Work out the finished part from the listing and answer in its coordinate system (mm). A direction names the side the tool comes from. Give positions to 0.01 mm unless a question says otherwise; leave off trailing zeros. Loops run counter-clockwise (first coordinate to the right, second up) from the corner with the lowest first, then second, coordinate; pieces in that order, holes last. Notation, with made-up numbers: (6, -39.5) - (31, -39.5) arc R22 cw to (31, -14.5) - close; hole circle Ø5 at (-35, 73.25). An arc over 180 degrees is marked (long way). One line per question, with ' | ' between items.
from build123d import *

# Parameters (mm, degrees)
CROQUIS1_R                 = 30.5
SALIENTE_EXTRUIR1_DEPTH    = 2.4
CROQUIS2_R                 = 2
CORTAR_EXTRUIR1_DEPTH      = 4
CORTAR_EXTRUIR3_START      = -4
CORTAR_EXTRUIR3_DEPTH      = 4
CORTAR_EXTRUIR5_START      = -4
CORTAR_EXTRUIR5_DEPTH      = 4
CORTAR_EXTRUIR6_DEPTH      = 10
CROQUIS10_R                = 2.5
CORTAR_EXTRUIR7_DEPTH      = 3
CORTAR_EXTRUIR8_DEPTH      = 44.200231628
CORTAR_EXTRUIR8_DEPTH_BACK = 44.200231628
CORTAR_EXTRUIR9_START      = -10
CORTAR_EXTRUIR9_DEPTH      = 10
REDONDEO1_R                = 1
CORTAR_EXTRUIR10_DEPTH     = 3


with BuildPart() as part:
    # Croquis1 → Saliente-Extruir1 (new body)
    with BuildSketch(Plane(origin=(0, 0, 0), x_dir=(1, 0, 0), z_dir=(0, 1, 0))):
        with Locations(Location((0, 0, 0), (0, 0, 270))):
            Circle(CROQUIS1_R)
    extrude(amount=SALIENTE_EXTRUIR1_DEPTH)

    # Croquis2 → Cortar-Extruir1 (cut)
    with BuildSketch(Plane(origin=(0, 2.4, 0), x_dir=(1, 0, 0), z_dir=(0, 1, 0))):
        with Locations(Location((0, 0, 0), (0, 0, 270))):
            Circle(CROQUIS2_R)
    extrude(amount=-CORTAR_EXTRUIR1_DEPTH, mode=Mode.SUBTRACT)

    # Croquis5 → Cortar-Extruir3 (cut)
    with BuildSketch(Plane(origin=(0, 2.4, 0), x_dir=(1, 0, 0), z_dir=(0, 1, 0)).offset(CORTAR_EXTRUIR3_START)):
        with BuildLine():
            Line((28.814059068, 5), (30.087372767, 5))
            ThreePointArc((30.087372767, 5), (29.556634924, 7.526973624), (28.814059068, 10))
            Line((28.814059068, 10), (24.814059068, 10))
            Line((24.814059068, 10), (24.814059068, 5))
            Line((24.814059068, 5), (28.814059068, 5))
        make_face()
        with BuildLine():
            Line((30.087372767, -5), (28.814059068, -5))
            Line((28.814059068, -5), (24.814059068, -5))
            Line((24.814059068, -5), (24.814059068, -10))
            Line((24.814059068, -10), (28.814059068, -10))
            ThreePointArc((28.814059068, -10), (29.556634924, -7.526973624), (30.087372767, -5))
        make_face()
        with BuildLine():
            Line((-24.814059068, 5), (-24.814059068, 10))
            Line((-24.814059068, 10), (-28.814059068, 10))
            ThreePointArc((-28.814059068, 10), (-29.556634924, 7.526973624), (-30.087372767, 5))
            Line((-30.087372767, 5), (-28.814059068, 5))
            Line((-28.814059068, 5), (-24.814059068, 5))
        make_face()
        with BuildLine():
            Line((-28.814059068, -10), (-24.814059068, -10))
            Line((-24.814059068, -10), (-24.814059068, -5))
            Line((-24.814059068, -5), (-28.814059068, -5))
            Line((-28.814059068, -5), (-30.087372767, -5))
            ThreePointArc((-30.087372767, -5), (-29.556634924, -7.526973624), (-28.814059068, -10))
        make_face()
    extrude(amount=CORTAR_EXTRUIR3_DEPTH, mode=Mode.SUBTRACT)

    # Croquis7 → Cortar-Extruir5 (cut)
    with BuildSketch(Plane(origin=(0, 2.4, 0), x_dir=(1, 0, 0), z_dir=(0, 1, 0)).offset(CORTAR_EXTRUIR5_START)):
        Polygon((1.428390211, 22.411430151), (-0.869743118, 20.483067322), (2.34419493, 16.652845106), (4.642328259, 18.581207935), align=None)
        with BuildLine():
            Line((-24.814059068, -10), (-28.814059068, -10))
            ThreePointArc((-28.814059068, -10), (0, -30.5), (28.814059068, -10))
            Line((28.814059068, -10), (24.814059068, -10))
            add(Edge.make_bspline(
                [(24.814059068, -10), (22.863263717, -9.657344338), (20.984021298, -8.980450277), (19.168992989, -8.065339906)],
                knots=[0, 0, 0, 0, 0.087850084, 0.087850084, 0.087850084, 0.087850084], degree=3))
            Line((19.168992989, -8.065339906), (11.455541673, 1.127193412))
            Line((11.455541673, 1.127193412), (9.248678515, -0.72458465))
            add(Edge.make_bspline(
                [(9.248678515, -0.72458465), (4.033234859, 4.116641048), (-0.646914404, 9.508508747), (-5.04935939, 12.080675515)],
                knots=[0.258799312, 0.258799312, 0.258799312, 0.258799312, 0.546435258, 0.546435258, 0.546435258, 0.546435258], degree=3))
            Line((-5.04935939, 12.080675515), (-0.757422911, 15.682037831))
            Line((-0.757422911, 15.682037831), (-7.828086618, 24.108526705))
            Line((-7.828086618, 24.108526705), (-17.020619935, 16.395075389))
            Line((-17.020619935, 16.395075389), (-13.66601447, 12.397212273))
            add(Edge.make_bspline(
                [(-13.66601447, 12.397212273), (-17.403465693, 9.897923685), (-21.056529869, 3.255841362), (-24.814059068, -10)],
                knots=[0.740637404, 0.740637404, 0.740637404, 0.740637404, 1, 1, 1, 1], degree=3))
        make_face()
        Polygon((14.685884661, 6.611763511), (12.387751331, 4.683400682), (15.60168938, 0.853178467), (17.899822709, 2.781541296), align=None)
    extrude(amount=CORTAR_EXTRUIR5_DEPTH, mode=Mode.SUBTRACT)

    # Croquis9 → Cortar-Extruir6 (cut)
    with BuildSketch(Plane(origin=(0, 2.4, 0), x_dir=(1, 0, 0), z_dir=(0, 1, 0))):
        Polygon((7.971418181, 14.613753061), (5.673284852, 12.685390231), (8.887222901, 8.855168016), (11.18535623, 10.783530845), align=None)
    extrude(amount=-CORTAR_EXTRUIR6_DEPTH, mode=Mode.SUBTRACT)

    # Croquis10 → Cortar-Extruir7 (cut)
    with BuildSketch(Plane(origin=(0, 2.4, 0), x_dir=(1, 0, 0), z_dir=(0, 1, 0))):
        with Locations(Location((12, 16, 0), (0, 0, 270))):
            Circle(CROQUIS10_R)
    extrude(amount=-CORTAR_EXTRUIR7_DEPTH, mode=Mode.SUBTRACT)

    # Croquis11 → Cortar-Extruir8 (cut, two sides: drawn at the far end of the back side and taken through both)
    with BuildSketch(Plane(origin=(0, 2.4, 0), x_dir=(1, 0, 0), z_dir=(0, 1, 0)).offset(-CORTAR_EXTRUIR8_DEPTH_BACK)):
        with BuildLine():
            Line((30.087372767, 5), (27.814059068, 5))
            Line((27.814059068, 5), (27.814059068, -5))
            Line((27.814059068, -5), (30.087372767, -5))
            ThreePointArc((30.087372767, -5), (30.5, 0), (30.087372767, 5))
        make_face()
        with BuildLine():
            ThreePointArc((28.814059068, 10), (28.341972277, 11.268655974), (27.814059068, 12.515115586))
            Line((27.814059068, 12.515115586), (27.814059068, 10))
            Line((27.814059068, 10), (28.814059068, 10))
        make_face()
        with BuildLine():
            Line((-27.814059068, -5), (-27.814059068, 5))
            Line((-27.814059068, 5), (-30.087372767, 5))
            ThreePointArc((-30.087372767, 5), (-30.5, 0), (-30.087372767, -5))
            Line((-30.087372767, -5), (-27.814059068, -5))
        make_face()
        with BuildLine():
            Line((-28.814059068, 10), (-27.814059068, 10))
            Line((-27.814059068, 10), (-27.814059068, 12.515115586))
            ThreePointArc((-27.814059068, 12.515115586), (-28.341972277, 11.268655974), (-28.814059068, 10))
        make_face()
    extrude(amount=CORTAR_EXTRUIR8_DEPTH + CORTAR_EXTRUIR8_DEPTH_BACK, mode=Mode.SUBTRACT)

    # Croquis12 → Cortar-Extruir9 (cut)
    with BuildSketch(Plane(origin=(0, 2.4, 0), x_dir=(1, 0, 0), z_dir=(0, 1, 0)).offset(CORTAR_EXTRUIR9_START)):
        with BuildLine():
            Line((-0.28585192, 30.498660441), (27.814059068, 11.545031156))
            Line((27.814059068, 11.545031156), (27.814059068, 12.515115586))
            ThreePointArc((27.814059068, 12.515115586), (16.440879495, 25.689442995), (-0.28585192, 30.498660441))
        make_face()
    extrude(amount=CORTAR_EXTRUIR9_DEPTH, mode=Mode.SUBTRACT)

    # Redondeo1
    redondeo1_edges = [part.edges().sort_by_distance(p)[0] for p in [
        (27.814059068, 1.2, -10),
        (-27.814059068, 1.2, -10),
    ]]
    fillet(redondeo1_edges, radius=REDONDEO1_R)

    # Croquis13 → Cortar-Extruir10 (cut)
    with BuildSketch(Plane(origin=(0, 2.4, 0), x_dir=(1, 0, 0), z_dir=(0, 1, 0))):
        Polygon((1.428390211, 22.411430151), (-0.869743118, 20.483067322), (-1.062579401, 20.712880655), (1.235553928, 22.641243484), align=None)
        Polygon((2.34419493, 16.652845106), (4.642328259, 18.581207935), (4.835164542, 18.351394602), (2.537031213, 16.423031773), align=None)
        Polygon((7.971418181, 14.613753061), (5.673284852, 12.685390231), (5.480448569, 12.915203564), (7.778581899, 14.843566393), align=None)
        Polygon((8.887222901, 8.855168016), (11.18535623, 10.783530845), (11.378192513, 10.553717512), (9.080059183, 8.625354683), align=None)
        Polygon((14.685884661, 6.611763511), (12.387751331, 4.683400682), (12.194915048, 4.913214015), (14.493048378, 6.841576844), align=None)
        Polygon((17.899822709, 2.781541296), (15.60168938, 0.853178467), (15.794525663, 0.623365134), (18.092658992, 2.551727963), align=None)
    extrude(amount=-CORTAR_EXTRUIR10_DEPTH, mode=Mode.SUBTRACT)


solid = part.part
1. Determine the mould class of faces 1 (the flat face through (-26, 1, 5)), 2 (the flat face through (0.07, 1.217, -21.664)), 3 (the flat face through (24.814, 1, 7)) for opening direction X: +X half, -X half, draft (parallel to the pull), parting line (faces both ways), or undercut.
Evaluation:
face 1: draft | face 2: undercut | face 3: +X half
2. Consider L1, parallel to X at y = 1.65, z = -16; L2, parallel to X at y = 0.4, z = -6; L3, parallel to Z at x = -16, y = 0.25. Determine where each line is inside the solid, lowest interval first.
Evaluation:
L1: -25.97 to -16.69, -1.02 to 9.5, 14.5 to 21.21 | L2: -24.81 to -18.83, 2.34 to 13.49, 15.2 to 24.81 | L3: -25.97 to -17.25, -15.18 to -10.26
3. Flat-ended cylindrical pins translate along their axes: pin 1 (1.2 mm diameter, centred on y = 1.5, z = 8.5, fed in from -X); pin 2 (0.7 mm diameter, centred on x = -26.5, y = 1, fed in from +Z); pin 3 (0.7 mm diameter, centred on x = 26, y = 1, fed in from -Z). Find the tip coordinate at first contact, or state that the pin passes through.
Evaluation:
pin 1: x = -24.81 | pin 2: z = 5 | pin 3: z = -13
4. Find section C-C on x = -6.5. Write down the section's boundary in (y, z), then the cut area to 3 significant figures.
Evaluation:
outline: (0, -29.8) - (2.4, -29.8) - (2.4, -22.53) - (0, -22.53) - close | area: 17.5 mm2
5. Which of the six approach directions +Z, -Z, +X, -X, +Y, -Y give full straight-line access (tool end or side, diameter ignored) to faces 4 (the flat face through (10.245, 1.217, -9.603)), 5 (the flat face through (26, 1, -10)), 6 (the flat face through (26, 1, 5)), 7 (the flat face through (-24.814, 1, -7)), 8 (the flat face through (15.366, 1.183, 3.533))?
Evaluation:
face 4: +Y, -Y | face 5: +X, +Y, -Y | face 6: +Z, +X, +Y, -Y | face 7: -X, +Y, -Y | face 8: +Z, +Y, -Y
6. Find section A-A on x = 16.5. Write down the section's boundary in (y, z).
Evaluation:
outline: (0, -19.18) - (2.4, -19.18) - (2.4, -4.45) - (0, -4.45) - close; (0, -1.22) - (2.4, -1.22) - (2.4, 4.88) - (0, 4.88) - close
7. Find section B-B on y = 0.4. State how many separate pieces and enclosed holes the cut face has, then the cut area to 3 significant figures.
Evaluation:
separate pieces: 1 | enclosed holes: 4 | area: 949 mm2
